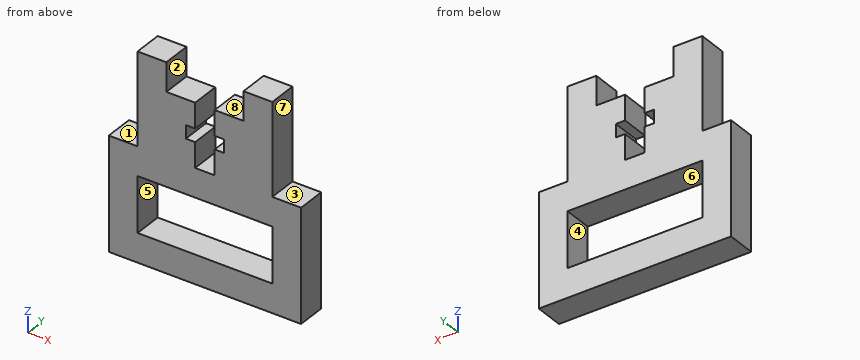
from build123d import *

# Parameters (mm, degrees)
SKETCH1_W           = 29.718
SKETCH1_H           = 12.192
BOSS_EXTRUDE1_DEPTH = 6.35


with BuildPart() as part:
    # Sketch1 → Boss-Extrude1 (new body)
    with BuildSketch(Plane(origin=(0, 0, 0), x_dir=(1, 0, 0), z_dir=(0, 1, 0))):
        Polygon((8.509, -26.416), (2.159, -26.416), (2.159, -20.881000021), (4.199999982, -20.881000021), (4.199999982, -17.980999979), (2.159, -17.980999979), (2.159, -12.446), (-2.159, -12.446), (-2.159, -17.980999979), (-4.199999982, -17.980999979), (-4.199999982, -20.881000021), (-2.159, -20.881000021), (-2.159, -26.416), (-8.509, -26.416), (-8.509, -32.766), (-14.859, -32.766), (-14.859, -26.416), (-14.859, -12.446), (-21.209, -12.446), (-21.209, 12.446), (21.209, 12.446), (21.209, -12.446), (14.859, -12.446), (14.859, -26.416), (14.859, -32.766), (8.509, -32.766), align=None)
        Rectangle(SKETCH1_W, SKETCH1_H, mode=Mode.SUBTRACT)
    extrude(amount=BOSS_EXTRUDE1_DEPTH)


solid = part.part
Part model, mm, in its own coordinate system. Face numbers are marked on the shaded views. A direction names the side the tool comes from. Give positions to 0.01 mm unless a question says otherwise; leave off trailing zeros. Write each loop counter-clockwise with the first axis right and the second up, starting at its lowest first coordinate (ties: lowest second). Pieces come first, ordered by that corner, then holes.
1) Pin check, flat tips, straight feed: pin 1 (3 mm diameter, centred on x = -5.5, y = 3, fed in from +Z); pin 2 (1.9 mm diameter, centred on x = 17.5, y = 4, fed in from +Z); pin 3 (2.5 mm diameter, centred on y = 2, z = 19.5, fed in from +X). Stop position of each tip, or through.
Resolved:
pin 1: stops at z = 26.42
pin 2: stops at z = 12.45
pin 3: stops at x = 14.86
2) Which spindle directions (+Z, -Z, +X, -X, +Y, -Y) get a long thin tool onto all of the face, cutting with end or side? Do the marked faces 1, 2, 3 and 4. Say none if no direction does.
Resolved:
face 1: +Z, -X, +Y, -Y
face 2: +Z, +Y, -Y
face 3: +Z, +X, +Y, -Y
face 4: +Y, -Y
3) Two-plate mould, pull along Z, no slides. Class the marked faces 5, 6, 7 and 8: released by +Z, released by -Z, zero draft, split by the parting line, or undercut.
Resolved:
face 5: undercut
face 6: undercut
face 7: zero draft
face 8: released by +Z
4) Cut at C-C on y = 5.25. Write the cut outline in (x, z).
Resolved:
outline: (-21.21, -12.45) - (21.21, -12.45) - (21.21, 12.45) - (14.86, 12.45) - (14.86, 32.77) - (8.51, 32.77) - (8.51, 26.42) - (2.16, 26.42) - (2.16, 20.88) - (4.2, 20.88) - (4.2, 17.98) - (2.16, 17.98) - (2.16, 12.45) - (-2.16, 12.45) - (-2.16, 17.98) - (-4.2, 17.98) - (-4.2, 20.88) - (-2.16, 20.88) - (-2.16, 26.42) - (-8.51, 26.42) - (-8.51, 32.77) - (-14.86, 32.77) - (-14.86, 12.45) - (-21.21, 12.45) - close; hole (-14.86, -6.1) - (14.86, -6.1) - (14.86, 6.1) - (-14.86, 6.1) - close
5) Probe L1, parallel to X at y = 3.5, z = 21.5; L2, parallel to Z at x = 5, y = 3; L3, parallel to X at y = 3.5, z = 6. List the from-to ranges inside material, lowest first.
Resolved:
L1: x = -14.86 to -2.16, 2.16 to 14.86
L2: z = -12.45 to -6.1, 6.1 to 26.42
L3: x = -21.21 to -14.86, 14.86 to 21.21
6) Cut at B-B on z = 23. Write the cut outline in (x, y), then the cut area to 3 significant figures.
Resolved:
outline: (-14.86, 0) - (-2.16, 0) - (-2.16, 6.35) - (-14.86, 6.35) - close; (2.16, 0) - (14.86, 0) - (14.86, 6.35) - (2.16, 6.35) - close
area: 161 mm2
7) Cut at A-A on x = 1. Write the cut outline in (y, z), then the cut area to 3 significant figures.
Resolved:
outline: (0, -12.45) - (6.35, -12.45) - (6.35, -6.1) - (0, -6.1) - close; (0, 6.1) - (6.35, 6.1) - (6.35, 12.45) - (0, 12.45) - close
area: 80.6 mm2
8) Cut at D-D on x = 15.5. Write the cut outline in (y, z), then the cut area to 3 significant figures.
Resolved:
outline: (0, -12.45) - (6.35, -12.45) - (6.35, 12.45) - (0, 12.45) - close
area: 158 mm2
